Geometry check sheet. Reference: the model listing, model coordinates, mm. A direction names the side the tool comes from. Coordinates: 2 decimals unless noted, no trailing zeros. Order: outer loops, then holes, each group sorted by start corner. A loop starts at its lowest first (then second) coordinate and runs counter-clockwise, first axis right, second up.
```python
from build123d import *

# Parameters (mm, degrees)
F1_DEPTH = 1020
F2_W     = 90
F2_H     = 100
F3_DEPTH = 25


with BuildPart() as f1:
    # F0 (on Top) → F1 (new body)
    with BuildSketch(Plane.XY):
        Polygon((7.455844, 18), (0, 0), (550, 0), (550, 18), align=None)
    extrude(amount=F1_DEPTH)

    # F2 (on Front) → F3 (cut)
    with BuildSketch(Plane.XZ):
        with Locations((505, 50)):
            Rectangle(F2_W, F2_H)
    extrude(amount=-F3_DEPTH, mode=Mode.SUBTRACT)


solid = f1.part
```
Item 1: Thickness scan on line 1 along Z through (x, y) = (514, 9.5); line 2 along X through (y, z) = (8, 912.5); line 3 along X through (y, z) = (9.75, 434). Record the ranges inside material, lowest first.
Item 2: Sectioned sample at A-A (y = 12.25). Record the cut outline in (x, z), and give its area (3 significant figures).
Item 3: Depth check by flat-ended pin: P1, Ø8, axis at y = 12.5, z = 137.5, coming from the -X side; P2, Ø6, axis at y = 7, z = 814.5, coming from the -X side. Enter the tip coordinate at first touch or a pass-through.
Item 4: Tool access check on faces 1 (the face through (283, 18, 503)), 2 (the face through (504, 9, 100)). Record the directions out of +Z, -Z, +X, -X, +Y, -Y that give a thin tool (end or side, any length) a straight path to the whole face; none if there is none.
Geometry check:
1. line 1: z = 100 to 1020
1. line 2: x = 3.31 to 550
1. line 3: x = 4.04 to 550
2. outline: (5.07, 0) - (460, 0) - (460, 100) - (550, 100) - (550, 1020) - (5.07, 1020) - close
2. area: 547,000 mm2
3. P1: stops at x = 3.52
3. P2: stops at x = 1.66
4. face 1: +Z, -Z, +X, -X, +Y
4. face 2: -Z, +X, +Y, -Y
